Study the drawing (mm; zero at the part's minimum x, y, z) and answer. A direction names the side the tool comes from. Round coordinates to 2 decimals unless told otherwise and drop trailing zeros. Loops run counter-clockwise (first coordinate to the right, second up) from the corner with the lowest first, then second, coordinate; pieces in that order, holes last. Notation, with made-up numbers: (80.5, 25) -> (123.5, 25) arc R17 ccw to (123.5, 31) -> close; hole circle Ø2 at (-12, -2). An arc over 180 degrees is marked (long way). Answer in a Markdown table with one row per item. Add a question column.
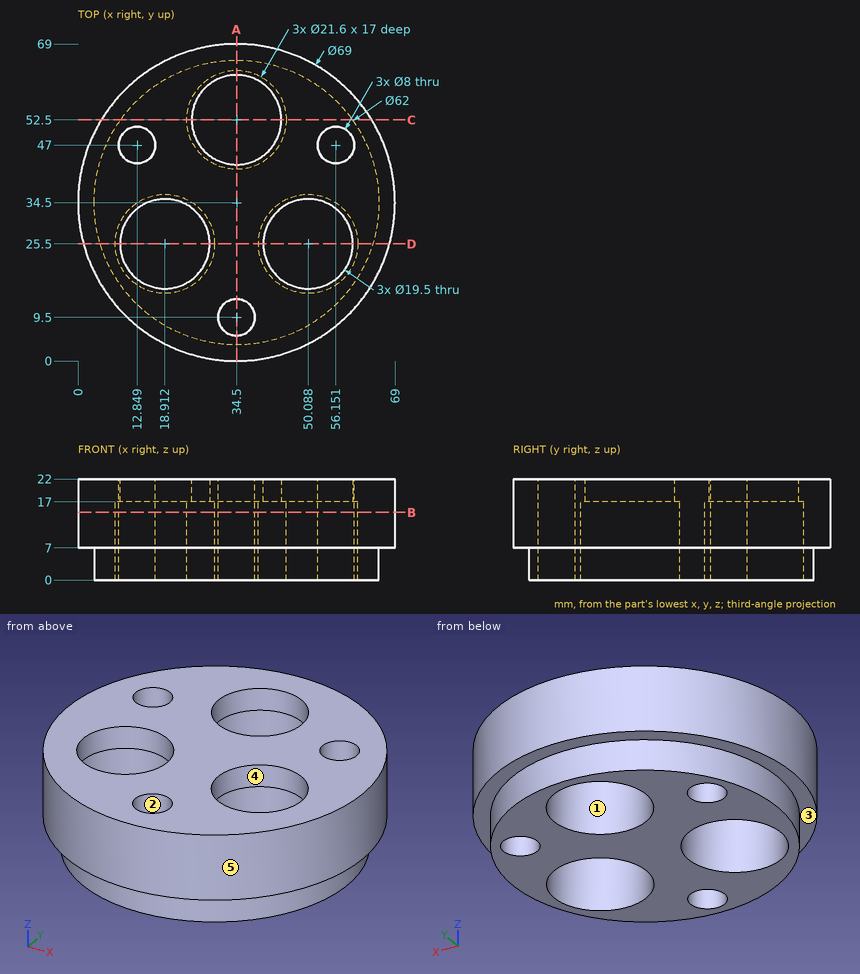
Item 1: Section B-B, the plane z = 14.75 is taken. Write down the section's boundary in (x, y), and give its area (3 significant figures).
Item 2: The mould has two halves that part along Y. Classify the marked faces 3, 4 and 5: +Y half, -Y half, draft (parallel to the pull), parting line (faces both ways), or undercut.
Item 3: Consider L1, parallel to Y at x = 34.5, z = 13.75; L2, parallel to Y at x = 34.5, z = 20.4; L3, parallel to X at y = 25.5, z = 9 (1 decimal). Determine where each line is inside the solid, lowest interval first. Write a range as from..to.
Item 4: Flat-ended cylindrical pins translate along their axes: P1, Ø12, axis at x = 17, z = 9, coming from the +Y side; P2, Ø15.5, axis at x = 34.5, y = 52.5, coming from the -Z side; P3, Ø17.5, axis at x = 45, y = 25.5, coming from the -Z side; P4, Ø3, axis at y = 17.5, z = 8.5, coming from the -X side. Find the tip coordinate at first contact, or state that the pin passes through.
Item 5: Section A-A, the plane x = 34.5 is taken. Write down the section's boundary in (y, z).
Item 6: Section D-D, the plane y = 25.5 is taken. Write down the section's boundary in (x, z) (1 decimal).
Item 7: For the marked faces 1 and 2, determine the directions among +Z, -Z, +X, -X, +Y, -Y from which every point of the face is accessible in a straight line to the end or side of a thin tool.
Item 8: Section C-C, the plane y = 52.5 is taken. Write down the section's boundary in (x, z).
Here are the results:
| question | item | result |
|---|---|---|
| 1 | outline | circle Ø69 at (34.5, 34.5); hole circle Ø21.6 at (18.91, 25.5); hole circle Ø8 at (12.85, 47); hole circle Ø21.6 at (34.5, 52.5); hole circle Ø8 at (34.5, 9.5); hole circle Ø21.6 at (50.09, 25.5); hole circle Ø8 at (56.15, 47) |
| 1 | area | 2,490 mm² |
| 2 | face 3 | draft |
| 2 | face 4 | undercut |
| 2 | face 5 | parting line |
| 3 | L1 | y = 0..5.5, 13.5..41.7, 63.3..69 |
| 3 | L2 | y = 0..5.5, 13.5..42.75, 62.25..69 |
| 3 | L3 | x = 1.2..8.1, 29.7..39.3, 60.9..67.8 |
| 4 | P1 | stops at y = 67.03 |
| 4 | P2 | passes through |
| 4 | P3 | stops at z = 0 |
| 4 | P4 | stops at x = 3.68 |
| 5 | outline | (0, 7) -> (3.5, 7) -> (3.5, 0) -> (5.5, 0) -> (5.5, 22) -> (0, 22) -> close; (13.5, 0) -> (41.7, 0) -> (41.7, 17) -> (42.75, 17) -> (42.75, 22) -> (13.5, 22) -> close; (62.25, 17) -> (63.3, 17) -> (63.3, 0) -> (65.5, 0) -> (65.5, 7) -> (69, 7) -> (69, 22) -> (62.25, 22) -> close |
| 6 | outline | (1.2, 7) -> (4.8, 7) -> (4.8, 0) -> (8.1, 0) -> (8.1, 17) -> (9.2, 17) -> (9.2, 22) -> (1.2, 22) -> close; (28.7, 17) -> (29.7, 17) -> (29.7, 0) -> (39.3, 0) -> (39.3, 17) -> (40.3, 17) -> (40.3, 22) -> (28.7, 22) -> close; (59.8, 17) -> (60.9, 17) -> (60.9, 0) -> (64.2, 0) -> (64.2, 7) -> (67.8, 7) -> (67.8, 22) -> (59.8, 22) -> close |
| 7 | face 1 | -Z |
| 7 | face 2 | +Z, -Z |
| 8 | outline | (5.07, 7) -> (9.26, 7) -> (9.26, 0) -> (23.7, 0) -> (23.7, 17) -> (24.75, 17) -> (24.75, 22) -> (5.07, 22) -> close; (44.25, 17) -> (45.3, 17) -> (45.3, 0) -> (59.74, 0) -> (59.74, 7) -> (63.93, 7) -> (63.93, 22) -> (44.25, 22) -> close |
